from build123d import *

# Parameters (mm, degrees)
SKETCH1_W             = 31.75
SKETCH1_H             = 9.525
BOSS_EXTRUDE1_DEPTH   = 3.175
F_8_CLEARANCE_HOLE1_D = 4.4958
SKETCH4_W             = 25.4
SKETCH4_H             = 15.875
BOSS_EXTRUDE2_DEPTH   = 3.175
SKETCH5_W             = 4.7625
SKETCH5_H             = 15.875
BOSS_EXTRUDE3_DEPTH   = 31.75
CUT_EXTRUDE1_DEPTH    = 68.445400371
LPATTERN1_COUNT       = 2
LPATTERN1_PITCH       = 20.6375


with BuildPart() as part:
    # Sketch1 → Boss-Extrude1 (new body)
    with BuildSketch(Plane(origin=(0, 0, 0), x_dir=(1, 0, 0), z_dir=(0, 1, 0))):
        Rectangle(SKETCH1_W, SKETCH1_H)
    extrude(amount=BOSS_EXTRUDE1_DEPTH)

    # #8 Clearance Hole1 (through all)
    with Locations(Plane(origin=(0, 3.175, 0), x_dir=(1, 0, 0), z_dir=(0, 1, 0))):
        with Locations((-7.9375, 0), (7.9375, 0)):
            Hole(F_8_CLEARANCE_HOLE1_D / 2)

    # Sketch4 → Boss-Extrude2 (add)
    with BuildSketch(Plane(origin=(0, 0, 0), x_dir=(1, 0, 0), z_dir=(0, 1, 0))):
        with Locations((-28.575, 0)):
            Rectangle(SKETCH4_W, SKETCH4_H)
    extrude(amount=BOSS_EXTRUDE2_DEPTH)

    # Sketch5 → Boss-Extrude3 (add)
    with BuildSketch(Plane(origin=(0, 3.175, 0), x_dir=(1, 0, 0), z_dir=(0, 1, 0))):
        with Locations((-38.89375, 0)):
            Rectangle(SKETCH5_W, SKETCH5_H)
    boss_extrude3 = extrude(amount=BOSS_EXTRUDE3_DEPTH)

    # Sketch7 → Cut-Extrude1 (cut, through all)
    with BuildSketch(Plane.ZY.offset(41.275)):
        with BuildLine():
            Line((6, 34.925), (6, 9.525))
            ThreePointArc((6, 9.525), (0, 3.525), (-6, 9.525))
            Line((-6, 9.525), (-6, 34.925))
            ThreePointArc((-6, 34.925), (0, 40.925), (6, 34.925))
        make_face()
    cut_extrude1 = extrude(amount=-CUT_EXTRUDE1_DEPTH, mode=Mode.SUBTRACT)

    # LPattern1: Boss-Extrude3, Cut-Extrude1 ×2
    with Locations(*[(i * LPATTERN1_PITCH, 0, 0) for i in range(1, LPATTERN1_COUNT)]):
        add(boss_extrude3)
        add(cut_extrude1, mode=Mode.SUBTRACT)


solid = part.part
Design review of the part built by this model. Coordinates are the model's own, in mm. A direction names the side the tool comes from. Round coordinates to 2 decimals unless told otherwise and drop trailing zeros. Write each loop counter-clockwise with the first axis right and the second up, starting at its lowest first coordinate (ties: lowest second). Pieces come first, ordered by that corner, then holes. Notation, with made-up numbers: (38.25, -34.75) - (66.25, -34.75) arc R22 ccw to (66.25, -15.75) - close; hole circle Ø9 at (55.25, 80). An arc over 180 degrees is marked (long way). Return JSON: item names as keys, results as strings. Group by question number.
Item 1: We need section A-A on z = 0. Give the number of separate pieces and of enclosed holes in the cut face, and give its area (3 significant figures).
Item 2: We need section D-D on x = 3.5. Write out the cut boundary in (y, z) (1 decimal), and give its area (3 significant figures).
Item 3: For probe 1 along Y at (x, z) = (-24, 0.5) (3 decimals), list the stretches that pass through material, from the lowest coordinate up. Write a range as [from, to].
Item 4: We need section C-C on z = -6.75. Write out the cut boundary in (x, y) (1 decimal), and give its area (3 significant figures).
Item 5: We need section B-B on y = 24.5. Write out the cut boundary in (x, z) (1 decimal), and give its area (3 significant figures).
Item 6: Machinability: for faces 1 (the face through (-20.638, 17, 7)), 2 (the face through (0, 2, 4.762)), 3 (the face through (-39, 22, -6)), 4 (the face through (0, 2, -4.762)), which of the approach directions +Z, -Z, +X, -X, +Y, -Y give a long, thin tool a straight path to every point of the face, cutting with its end or side? Answer none if there is none.
Item 7: Insertion check: P1, Ø5, axis at x = -25.5, z = -1.5, coming from the +Y side (3 decimals); P2, Ø2.5, axis at x = 5, y = 1.5, coming from the +Z side; P3, Ø6, axis at x = -12, y = 24.5, coming from the +Z side; P4, Ø3.5, axis at x = -5, y = 2, coming from the -Z side. Each pin has a flat end and moves straight along its axis. Give the tip position at first contact, or say it passes through.
Item 8: The part is to be moulded in two halves that separate along Z. For faces 5 (the face through (-38.927, 3.526, 0.132)), 6 (the face through (-37, 17, 7.938)), 7 (the face through (-10.08, 1.57, -0.68)), 8 (the face through (-19, 0, 0)), say which applies: pulls with the +Z half, pulls with the -Z half, needs draft (parallel to the pull), parting line crosses it, or undercut.
Model answer:
{
 "1": {"separate pieces": "3", "enclosed holes": "0", "area": "156 mm²"},
 "2": {"outline": "(0, -4.8) - (3.2, -4.8) - (3.2, 4.8) - (0, 4.8) - close", "area": "30.2 mm²"},
 "3": {"probe 1": "y = [0, 3.175]"},
 "4": {"outline": "(-41.3, 0) - (-15.9, 0) - (-15.9, 34.9) - (-20.6, 34.9) - (-20.6, 3.2) - (-36.5, 3.2) - (-36.5, 34.9) - (-41.3, 34.9) - close", "area": "383 mm²"},
 "5": {"outline": "(-41.3, -7.9) - (-36.5, -7.9) - (-36.5, -6) - (-41.3, -6) - close; (-41.3, 6) - (-36.5, 6) - (-36.5, 7.9) - (-41.3, 7.9) - close; (-20.6, -7.9) - (-15.9, -7.9) - (-15.9, -6) - (-20.6, -6) - close; (-20.6, 6) - (-15.9, 6) - (-15.9, 7.9) - (-20.6, 7.9) - close", "area": "36.9 mm²"},
 "6": {"face 1": "+Z, -Z, +Y", "face 2": "+Z, +X, +Y, -Y", "face 3": "+X, -X, +Y", "face 4": "-Z, +X, +Y, -Y"},
 "7": {"P1": "stops at y = 3.175", "P2": "stops at z = 4.76", "P3": "passes through", "P4": "stops at z = -4.76"},
 "8": {"face 5": "undercut", "face 6": "pulls with the +Z half", "face 7": "undercut", "face 8": "needs draft"}
}
